from build123d import *

# Parameters (mm, degrees)
EXTRUDE_180_DEPTH      = 8
EXTRUDE_START          = 8
SKETCH_2_W             = 6
SKETCH_2_H             = 4
EXTRUDE_457_DEPTH      = 36
EXTRUDE_START_2        = 44
EXTRUDE_180_2_DEPTH    = 3
SKETCH_4_R             = 20
SKETCH_4_R_2           = 4
EXTRUDE_692_DEPTH      = 3
EXTRUDE_745_DEPTH      = 3
EXTRUDE_1_DEPTH        = 3
EXTRUDE_Y_1_DEPTH      = 3
EXTRUDE_1_2_DEPTH      = 3
EXTRUDE_Y_1_2_DEPTH    = 3
CUT_EXTRUDE_START      = 44
CUT_EXTRUDE_1134_DEPTH = 3
SKETCH_11_R            = 5
EXTRUDE_1203_DEPTH     = 3
EXTRUDE_1416_DEPTH     = 8
SKETCH_13_R            = 1.6
CUT_EXTRUDE_1487_DEPTH = 3
SKETCH_14_R            = 1.6
CUT_EXTRUDE_1548_DEPTH = 8
CUT_EXTRUDE_START_2    = 8
SKETCH_15_W            = 600
SKETCH_15_H            = 600
CUT_EXTRUDE_1608_DEPTH = 60
F_2MM_DEPTH            = 8
SKETCH_17_R            = 5
EXTRUDE_M3_DEPTH       = 8
SKETCH_18_R            = 5
EXTRUDE_3_DEPTH        = 8
SKETCH_19_R            = 5
EXTRUDE_4_DEPTH        = 8
SKETCH_20_R            = 1.6
CUT_EXTRUDE_M3_DEPTH   = 8
F_40MM_4MM_D6P2_START  = 4
SKETCH_21_R            = 3.1
F_40MM_4MM_D6P2_DEPTH  = 4
R3P9_R                 = 3.9
F_2MM_0_2_START        = 2
SKETCH_22_W            = 600
SKETCH_22_H            = 600
F_2MM_0_2_DEPTH        = 8
FILLET_4_R             = 1.4


with BuildPart() as part:
    # 草图1 → Extrude 180 (new body)
    with BuildSketch(Plane.XY):
        Polygon((0, -115), (35.536954353, -109.371499374), (70.801069662, -90.621236665), (96.447115314, -62.633489027), (111.081470023, -29.764190187), (115, 0), (111.081470023, 29.764190187), (96.447115314, 62.633489027), (70.801069662, 90.621236665), (35.536954353, 109.371499374), (0, 115), (0, 111), (34.300886376, 105.567273309), (68.338423761, 87.46919365), (93.092433042, 60.454932887), (107.217766718, 28.728914006), (111, 0), (107.217766718, -28.728914006), (93.092433042, -60.454932887), (68.338423761, -87.46919365), (34.300886376, -105.567273309), (0, -111), align=None)
    extrude(amount=EXTRUDE_180_DEPTH)

    # 草图2 → Extrude 457 (add)
    with BuildSketch(Plane.XY.offset(EXTRUDE_START)):
        Polygon((35.584965419, -103.047126287), (37.439067386, -108.753465385), (33.634841321, -109.989533363), (31.780739354, -104.283194265), align=None)
        with Locations((112, 0)):
            Rectangle(SKETCH_2_W, SKETCH_2_H)
        Polygon((31.780739354, 104.283194265), (33.634841321, 109.989533363), (37.439067386, 108.753465385), (35.584965419, 103.047126287), align=None)
    extrude(amount=EXTRUDE_457_DEPTH)

    # 草图3 → Extrude 180 2 (add)
    with BuildSketch(Plane.XY.offset(EXTRUDE_START_2)):
        Polygon((0, -115), (35.536954353, -109.371499374), (70.801069662, -90.621236665), (96.447115314, -62.633489027), (111.081470023, -29.764190187), (115, 0), (111.081470023, 29.764190187), (96.447115314, 62.633489027), (70.801069662, 90.621236665), (35.536954353, 109.371499374), (0, 115), (0, 109), (33.682852387, 103.665160276), (67.10710081, 85.893172143), (91.415091906, 59.365654817), (105.285915066, 28.211275916), (109, 0), (105.285915066, -28.211275916), (91.415091906, -59.365654817), (67.10710081, -85.893172143), (33.682852387, -103.665160276), (0, -109), align=None)
    extrude(amount=EXTRUDE_180_2_DEPTH)



with BuildPart() as body_2:
    # 草图4 → Extrude 692 (new body)
    with BuildSketch(Plane.XY.offset(EXTRUDE_START_2)):
        Circle(SKETCH_4_R)
        Circle(SKETCH_4_R_2, mode=Mode.SUBTRACT)
    extrude(amount=EXTRUDE_692_DEPTH)


with BuildPart() as part_1:
    add(part.part)

    add(body_2.part)  # Extrude 745 merges body 2
    # 草图5 → Extrude 745 (add)
    with BuildSketch(Plane.XY.offset(EXTRUDE_START_2)):
        Polygon((17, -9), (113, -2.5), (113, 2.5), (17, 9), align=None)
    extrude(amount=EXTRUDE_745_DEPTH)

    # 草图6 → Extrude 1 (add)
    with BuildSketch(Plane.XY.offset(EXTRUDE_START_2)):
        Polygon((-5.736735419, -8.734652509), (31.330903272, -107.096180364), (26.669096728, -108.903819636), (-12.263264581, -11.265347491), align=None)
    extrude(amount=EXTRUDE_1_DEPTH)

    # 草图7 → Extrude Y__-1 (add)
    with BuildSketch(Plane.XY.offset(EXTRUDE_START_2)):
        Polygon((60.213265383, 1.279918343), (91.234949037, -66.240061243), (87.165050963, -68.159938757), (54.786734617, -1.279918343), align=None)
    extrude(amount=EXTRUDE_Y_1_DEPTH)

    # 草图8 → Extrude 1 2 (add)
    with BuildSketch(Plane.XY.offset(EXTRUDE_START_2)):
        Polygon((-12.263264581, 11.265347491), (26.669096728, 108.903819636), (31.330903272, 107.096180364), (-5.736735419, 8.734652509), align=None)
    extrude(amount=EXTRUDE_1_2_DEPTH)

    # 草图9 → Extrude Y__1 2 (add)
    with BuildSketch(Plane.XY.offset(EXTRUDE_START_2)):
        Polygon((54.786734617, 1.279918343), (87.165050963, 68.159938757), (91.234949037, 66.240061243), (60.213265383, -1.279918343), align=None)
    extrude(amount=EXTRUDE_Y_1_2_DEPTH)

    # 草图10 → Cut-Extrude 1134 (cut)
    with BuildSketch(Plane.XY.offset(CUT_EXTRUDE_START)):
        Polygon((18, -4.5), (18, 4.5), (80.33, 0), align=None)
    extrude(amount=CUT_EXTRUDE_1134_DEPTH, mode=Mode.SUBTRACT)

    # 草图11 → Extrude 1203 (add)
    with BuildSketch(Plane.XY.offset(EXTRUDE_START_2)):
        with Locations((0, 112)):
            Circle(SKETCH_11_R)
        with Locations((0, -112)):
            Circle(SKETCH_11_R)
    extrude(amount=EXTRUDE_1203_DEPTH)

    # 草图12 → Extrude 1416 (add)
    with BuildSketch(Plane.XY):
        Polygon((-5, -107), (5, -107), (5, -116.208077798), (0, -117), (-3, -115), (-5, -112), align=None)
        Polygon((-5, 107), (5, 107), (5, 116.208077798), (0, 117), (-3, 115), (-5, 112), align=None)
    extrude(amount=EXTRUDE_1416_DEPTH)

    # 草图13 → Cut-Extrude 1487 (cut)
    with BuildSketch(Plane.XY.offset(CUT_EXTRUDE_START)):
        with Locations((13.435028843, 0)):
            Circle(SKETCH_13_R)
        with Locations((-13.435028843, 0)):
            Circle(SKETCH_13_R)
        with Locations((0, 13.435028843)):
            Circle(SKETCH_13_R)
        with Locations((0, -13.435028843)):
            Circle(SKETCH_13_R)
        with Locations((0, 112)):
            Circle(SKETCH_13_R)
        with Locations((0, -112)):
            Circle(SKETCH_13_R)
    extrude(amount=CUT_EXTRUDE_1487_DEPTH, mode=Mode.SUBTRACT)

    # 草图14 → Cut-Extrude 1548 (cut)
    with BuildSketch(Plane.XY):
        with Locations((0, 112)):
            Circle(SKETCH_14_R)
        with Locations((0, -112)):
            Circle(SKETCH_14_R)
    extrude(amount=CUT_EXTRUDE_1548_DEPTH, mode=Mode.SUBTRACT)

    # 草图15 → Cut-Extrude 1608 (cut)
    with BuildSketch(Plane.XY.offset(CUT_EXTRUDE_START_2)):
        Rectangle(SKETCH_15_W, SKETCH_15_H)
    extrude(amount=CUT_EXTRUDE_1608_DEPTH, mode=Mode.SUBTRACT)

    # 草图16 → 外圈径向加厚2mm (add)
    with BuildSketch(Plane.XY):
        Polygon((0, -117), (36.154988342, -111.273612407), (72.032392613, -92.197258172), (98.12445645, -63.722767097), (113.013321676, -30.281828277), (117, 0), (113.013321676, 30.281828277), (98.12445645, 63.722767097), (72.032392613, 92.197258172), (36.154988342, 111.273612407), (0, 117), (0, 114), (35.227937359, 108.420442858), (70.185408187, 89.833225911), (95.608444746, 62.088849992), (110.115544197, 29.505371142), (114, 0), (110.115544197, -29.505371142), (95.608444746, -62.088849992), (70.185408187, -89.833225911), (35.227937359, -108.420442858), (0, -114), align=None)
    extrude(amount=F_2MM_DEPTH)

    # 草图17 → M3铝柱下定位耳 (add)
    with BuildSketch(Plane.XY):
        with Locations((35.227937359, -108.420442858)):
            Circle(SKETCH_17_R)
    extrude(amount=EXTRUDE_M3_DEPTH)

    # 草图18 → 凸台-拉伸3 (add)
    with BuildSketch(Plane.XY):
        with Locations((114, 0)):
            Circle(SKETCH_18_R)
    extrude(amount=EXTRUDE_3_DEPTH)

    # 草图19 → 凸台-拉伸4 (add)
    with BuildSketch(Plane.XY):
        with Locations((35.227937359, 108.420442858)):
            Circle(SKETCH_19_R)
    extrude(amount=EXTRUDE_4_DEPTH)

    # 草图20 → 三处M3下层固定孔 (cut)
    with BuildSketch(Plane.XY):
        with Locations((35.227937359, -108.420442858)):
            Circle(SKETCH_20_R)
        with Locations((114, 0)):
            Circle(SKETCH_20_R)
        with Locations((35.227937359, 108.420442858)):
            Circle(SKETCH_20_R)
    extrude(amount=CUT_EXTRUDE_M3_DEPTH, mode=Mode.SUBTRACT)

    # 草图21 → 40mm铝柱沉座_深4mm_D6p2 (cut)
    with BuildSketch(Plane.XY.offset(F_40MM_4MM_D6P2_START)):
        with Locations((35.227937359, -108.420442858)):
            Circle(SKETCH_21_R)
        with Locations((114, 0)):
            Circle(SKETCH_21_R)
        with Locations((35.227937359, 108.420442858)):
            Circle(SKETCH_21_R)
    extrude(amount=F_40MM_4MM_D6P2_DEPTH, mode=Mode.SUBTRACT)

    # 下端耳外缘圆角_R3p9_轮廓内收
    r3p9_edges = [part_1.edges().sort_by_distance(p)[0] for p in [
        (-5, -112, 4),
        (-3, -115, 4),
        (0, -117, 4),
        (-5, 112, 4),
        (0, 117, 4),
        (-3, 115, 4),
    ]]
    fillet(r3p9_edges, radius=R3P9_R)

    # 草图22 → 统一2mm板厚_下层保留0至2 (cut)
    with BuildSketch(Plane.XY.offset(F_2MM_0_2_START)):
        Rectangle(SKETCH_22_W, SKETCH_22_H)
    extrude(amount=F_2MM_0_2_DEPTH, mode=Mode.SUBTRACT)

    # 圆角4
    fillet_4_edges = [part_1.edges().sort_by_distance(p)[0] for p in [
        (5, 110.208077798, 1),
        (5, 107, 1),
        (-5, 107, 1),
        (-5, -107, 1),
        (5, -107, 1),
        (5, -110.208077798, 1),
    ]]
    fillet(fillet_4_edges, radius=FILLET_4_R)


solid = part_1.part
Design review of the part built by this model. Coordinates are the model's own, in mm. A direction names the side the tool comes from. Round coordinates to 2 decimals unless told otherwise and drop trailing zeros. Write each loop counter-clockwise with the first axis right and the second up, starting at its lowest first coordinate (ties: lowest second). Pieces come first, ordered by that corner, then holes.
Item 1: Consider section B-B on x = 59. Give the boundary of the cut face in (y, z), and give its area (3 significant figures).
Item 2: For pin 1 Ø3.5 at (x, y) = (114, 0) entering from +Z; pin 2 Ø1 at (x, z) = (-1, 1.5) entering from -Y, all flat-tipped, find the tip position at first contact; note any pin that passes through.
Item 3: For faces 1 (the flat face through (80.5, 74.2, 1)), 2 (the flat face through (105.465, -47.236, 0.986)), list the 3-axis set-ups (+Z, -Z, +X, -X, +Y, -Y) from which the entire face can be reached by the end or side of a thin tool; tool diameter is ignored.
Item 4: Consider section C-C on z = 1.4. Count the separate pieces of the cut face and the enclosed holes in it, and give its area (3 significant figures).
Item 5: Wall thickness on L1, parallel to Y at x = 0, z = 1.3; L2, parallel to Y at x = 96, z = 1.15; L3, parallel to Y at x = 41.5, z = 0.8: over which ranges is each line inside the solid? List them lowest first.
Item 6: Consider section D-D on y = 71. Give the boundary of the cut face in (x, z), and give its area (3 significant figures).
Item 7: Draft analysis for pull direction Y (two halves, no side actions). For faces 3 (the flat face through (80.89, -73.77, 0.99)), 4 (the flat face through (84.896, -78.159, 0.986)), 5 (the flat face through (85.26, 77.76, 0.99)), 6 (the flat face through (100.06, 44.81, 0.99)), state which applies: released by +Y, released by -Y, zero draft, split by the parting line, or undercut.
Item 8: Consider section A-A on x = 81.5. Give the boundary of the cut face in (y, z), and give its area (3 significant figures).
Check values:
1. outline: (-99.13, 0) - (-92.43, 0) - (-92.43, 2) - (-99.13, 2) - close; (92.43, 0) - (99.13, 0) - (99.13, 2) - (92.43, 2) - close
1. area: 26.8 mm2
2. pin 1: stops at z = 2
2. pin 2: stops at y = -116.55
3. face 1: +Z, -Z, -X
3. face 2: +Z, -Z, +X, -Y
4. separate pieces: 1
4. enclosed holes: 5
4. area: 2,260 mm2
5. L1: y = -116.71 to -113.6, -110.4 to -107, 107 to 110.4, 113.6 to 116.71
5. L2: y = -66.04 to -53.92, 53.92 to 66.04
5. L3: y = -108.43 to -101.74, 101.74 to 108.43
6. outline: (83.43, 0) - (91.46, 0) - (91.46, 2) - (83.43, 2) - close
6. area: 16.1 mm2
7. face 3: undercut
7. face 4: released by -Y
7. face 5: released by +Y
7. face 6: undercut
8. outline: (-81.87, 0) - (-73.11, 0) - (-73.11, 2) - (-81.87, 2) - close; (73.11, 0) - (81.87, 0) - (81.87, 2) - (73.11, 2) - close
8. area: 35.0 mm2
